Check sheet for the drawn part. Datum: minimum x, y, z corner. Units: mm. A direction names the side the tool comes from. Give positions to 0.01 mm unless a question says otherwise; leave off trailing zeros. Write each loop counter-clockwise with the first axis right and the second up, starting at its lowest first coordinate (ties: lowest second). Pieces come first, ordered by that corner, then holes. Notation, with made-up numbers: (37, 68) -> (96, 68) arc R28 ccw to (96, 94) -> close; hole circle Ø4 at (-4, 65.25). An arc over 180 degrees is marked (long way). Use CSV: the item, a comma, the result in double quotes. Start each with the question number.
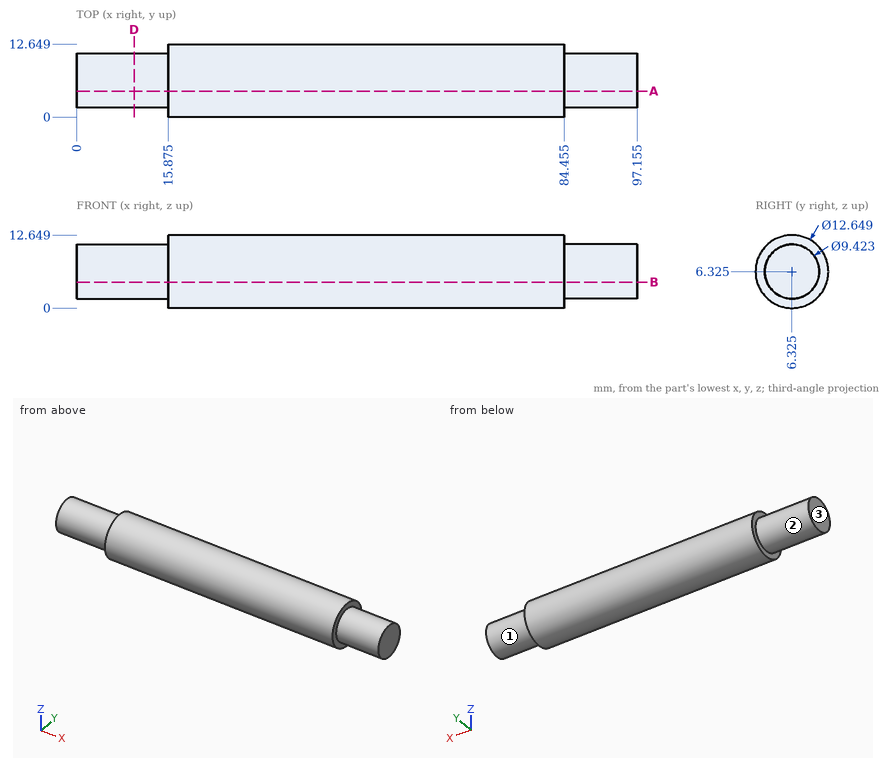
(1) Section check D-D on x = 10. Record the cut outline in (y, z) (1 decimal).
(2) Section check A-A on y = 4.5. Record the cut outline in (x, z) (1 decimal).
(3) Go/stop test with flat-tipped pins: pin 1 (3 mm diameter, centred on y = 5.5, z = 7, fed in from -X); pin 2 (2 mm diameter, centred on x = 23.5, y = 8, fed in from +Z); pin 3 (1.5 mm diameter, centred on x = 72.5, z = 3, fed in from +Y); pin 4 (2 mm diameter, centred on x = 20, y = 4, fed in from -Z). Record where each tip stops, or that it passes through.
(4) Set-up check for the marked faces 1, 2 and 3: record each of +Z, -Z, +X, -X, +Y, -Y from which the full face is reachable in a straight line by a thin tool's end or side.
(5) Thickness scan on line 1 (X direction, y = 1, z = 7) (1 decimal); line 2 (Z direction, x = 80.5, y = 6); line 3 (Z direction, x = 52, y = 7.5). Record the ranges inside material, lowest first. Write a range as from..to.
Data:
1,outline,"circle Ø9.4 at (6.3, 6.3)"
2,outline,"(0, 2) -> (15.9, 2) -> (15.9, 0.3) -> (84.5, 0.3) -> (84.5, 2) -> (97.2, 2) -> (97.2, 10.7) -> (84.5, 10.7) -> (84.5, 12.4) -> (15.9, 12.4) -> (15.9, 10.7) -> (0, 10.7) -> close"
3,pin 1,"stops at x = 0"
3,pin 2,"stops at z = 12.61"
3,pin 3,"stops at y = 12.1"
3,pin 4,"stops at z = 0.14"
4,face 1,"+X"
4,face 2,"-X"
4,face 3,"+Z, -Z, -X, +Y, -Y"
5,line 1,"x = 15.9..84.5"
5,line 2,"z = 0.01..12.64"
5,line 3,"z = 0.11..12.54"
